Check sheet for the modelled part. Datum: model origin and axes. Units: mm. A direction names the side the tool comes from. Round coordinates to 2 decimals unless told otherwise and drop trailing zeros. Write each loop counter-clockwise with the first axis right and the second up, starting at its lowest first coordinate (ties: lowest second). Pieces come first, ordered by that corner, then holes. Notation, with made-up numbers: (-10.75, 33) -> (9.25, 33) arc R23 cw to (9.25, 46) -> close; hole circle Ø11 at (21, -20). An arc over 180 degrees is marked (long way). Use one line per item in the form item = value. Start each with the question number.
```python
from build123d import *

# Parameters (mm, degrees)
BOSS_EXTRUDE1_DEPTH = 6.539992
SKETCH2_R           = 1.25000004
CUT_EXTRUDE1_DEPTH  = 5.08


with BuildPart() as part:
    # Sketch1 → Boss-Extrude1 (new body)
    with BuildSketch(Plane.XY):
        Polygon((-10.594624819, 2.728309468), (-10.24995918, 2.999994), (-9.905293541, 2.728309468), (-9.503891011, 2.905743672), (-9.237618872, 2.55687975), (-8.804701048, 2.628914782), (-8.633553268, 2.224791874), (-8.196321969, 2.186901508), (-8.131052392, 1.752912142), (-7.716980469, 1.60747717), (-7.761690222, 1.170890494), (-7.396795337, 0.927049129), (-7.548675142, 0.515297489), (-7.255884983, 0.188371182), (-7.505391673, -0.172673551), (-7.303103322, -0.562142819), (-7.634559474, -0.849794878), (-7.535483452, -1.27733532), (-7.928062458, -1.473520467), (-7.938424075, -1.912268145), (-8.367458751, -2.004659346), (-8.48660695, -2.427046129), (-8.925139471, -2.409838105), (-9.145587731, -2.789323879), (-9.566063484, -2.663597874), (-9.873960231, -2.976338151), (-10.24995918, -2.749993992), (-10.625958129, -2.976338151), (-10.933854876, -2.663597874), (-11.354330629, -2.789323879), (-11.574778889, -2.409838105), (-12.01331141, -2.427046129), (-12.132459609, -2.004659346), (-12.561494285, -1.912268145), (-12.571855902, -1.473520467), (-12.964434908, -1.27733532), (-12.865358886, -0.849794878), (-13.196815038, -0.562142819), (-12.994526687, -0.172673551), (-13.244033377, 0.188371182), (-12.951243218, 0.515297489), (-13.103123023, 0.927049129), (-12.738228138, 1.170890494), (-12.782937891, 1.60747717), (-12.368865968, 1.752912142), (-12.303596391, 2.186901508), (-11.866365092, 2.224791874), (-11.695217312, 2.628914782), (-11.262299488, 2.55687975), (-10.996027349, 2.905743672), align=None)
    extrude(amount=BOSS_EXTRUDE1_DEPTH)

    # Sketch2 → Cut-Extrude1 (cut)
    with BuildSketch(Plane.XY.offset(6.539992)):
        with Locations((-10.24995918, 0)):
            Circle(SKETCH2_R)
    extrude(amount=-CUT_EXTRUDE1_DEPTH, mode=Mode.SUBTRACT)


solid = part.part
```
1. Sectioned sample at C-C (y = -2.2). Enter the section's corners in (x, z).
2. Depth check by flat-ended pin: pin 1 (3 mm diameter, centred on y = 2, z = 1.5, fed in from -X); pin 2 (1.3 mm diameter, centred on x = -10, y = 0, fed in from +Z). Enter the tip coordinate at first touch or a pass-through.
3. Sectioned sample at A-A (y = 0). Enter the section's corners in (x, z).
4. Tool access check on faces 1 (the face through (-10, 0, 0)), 2 (the face through (-10, 0, 1.46)). Record the directions out of +Z, -Z, +X, -X, +Y, -Y that give a thin tool (end or side, any length) a straight path to the whole face; none if there is none.
5. Sectioned sample at B-B (y = 2.1). Enter the section's corners in (x, z), and give its area (3 significant figures).
6. Mould release check, pull along X, two halves, no side actions. Record for faces 3 (the face through (-12, 0, 6.54)), 4 (the face through (-9, 0, 4)): +X half, -X half, draft (parallel to the pull), parting line (faces both ways), or undercut.
7. Scan lines: probe 1 along Y at (x, z) = (-11.2, 4.25); probe 2 along Y at (x, z) = (-10.75, 1.75); probe 3 along X at (y, z) = (-1.85, 1.25). Record each from-to range of solid material in increasing order.
Returned:
q1.outline = (-12.08, 0) -> (-8.42, 0) -> (-8.42, 6.54) -> (-12.08, 6.54) -> close
q2.pin_1 = -13.1
q2.pin_2 = 1.46
q3.outline = (-13.11, 0) -> (-7.39, 0) -> (-7.39, 6.54) -> (-9, 6.54) -> (-9, 1.46) -> (-11.5, 1.46) -> (-11.5, 6.54) -> (-13.11, 6.54) -> close
q4.face_1 = -Z, +X, -X, +Y, -Y
q4.face_2 = +Z
q5.outline = (-12.32, 0) -> (-8.18, 0) -> (-8.18, 6.54) -> (-12.32, 6.54) -> close
q5.area = 27.0 mm^2
q6.face_3 = draft
q6.face_4 = undercut
q7.probe_1 = -2.74 to -0.81, 0.81 to 2.64
q7.probe_2 = -2.85 to -1.15, 1.15 to 2.8
q7.probe_3 = -12.56 to -7.94
